The drawing under review shows one solid part. Ordinate dimensions are in mm from its lowest x, y, z. Round coordinates to 2 decimals unless told otherwise and drop trailing zeros. Write each loop counter-clockwise with the first axis right and the second up, starting at its lowest first coordinate (ties: lowest second). Pieces come first, ordered by that corner, then holes.
Item 1: Add section A-A (x = 50.8). Give the boundary of the cut face in (y, z), plus the area to 3 significant figures.
Item 2: Add section C-C (y = 14). Give the boundary of the cut face in (x, z).
Item 3: To check wall thickness, follow L1, parallel to X at y = 14.5, z = 59; L2, parallel to Z at x = 60, y = 6. State the ranges of each line that lie inside material, in increasing order.
Item 4: Clearance check with flat-ended pins moving along their axes: pin 1 Ø8 at (x, z) = (50.8, 50.8) entering from -Y; pin 2 Ø1 at (y, z) = (8, 90.5) entering from -X; pin 3 Ø10 at (y, z) = (6, 11) entering from +X; pin 4 Ø2 at (x, y) = (17.5, 10) entering from +Z. State where each tip first meets the part, or that it passes through.
Item 5: Add section B-B (z = 50.8). Give the boundary of the cut face in (x, y).
Item 6: Add section D-D (x = 7.5). Give the boundary of the cut face in (y, z), plus the area to 3 significant figures.
Item 7: Draft analysis for pull direction Z (two halves, no side actions). For the marked faces 1, 2 and 3, state which applies: +Z half, -Z half, draft (parallel to the pull), parting line (faces both ways), or undercut.
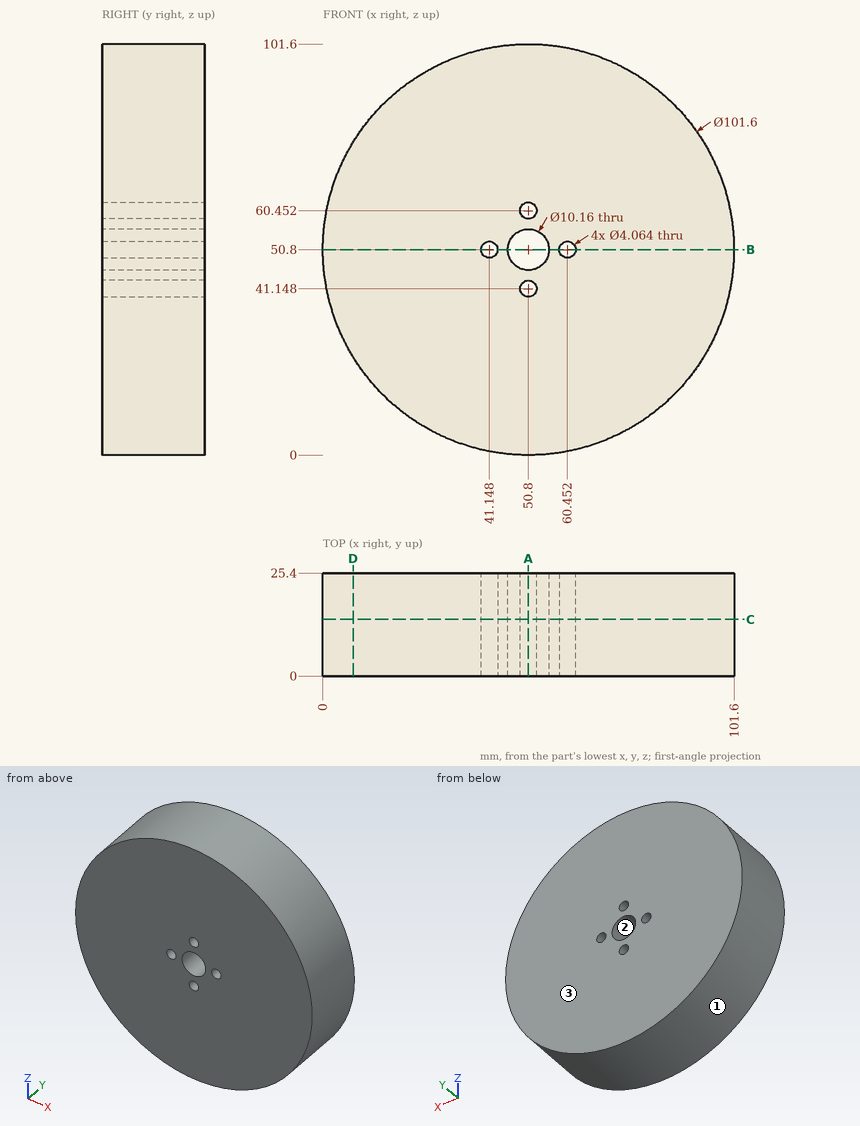
Numbers:
1. outline: (0, 0) - (25.4, 0) - (25.4, 39.12) - (0, 39.12) - close; (0, 43.18) - (25.4, 43.18) - (25.4, 45.72) - (0, 45.72) - close; (0, 55.88) - (25.4, 55.88) - (25.4, 58.42) - (0, 58.42) - close; (0, 62.48) - (25.4, 62.48) - (25.4, 101.6) - (0, 101.6) - close
1. area: 2,120 mm2
2. outline: circle Ø101.6 at (50.8, 50.8); hole circle Ø4.06 at (41.15, 50.8); hole circle Ø10.16 at (50.8, 50.8); hole circle Ø4.06 at (50.8, 41.15); hole circle Ø4.06 at (50.8, 60.45); hole circle Ø4.06 at (60.45, 50.8)
3. L1: x = 0.67 to 49.38, 52.22 to 100.93
3. L2: z = 0.84 to 48.82, 52.78 to 100.76
4. pin 1: passes through
4. pin 2: stops at x = 18.49
4. pin 3: stops at x = 87.81
4. pin 4: stops at z = 90.01
5. outline: (0, 0) - (39.12, 0) - (39.12, 25.4) - (0, 25.4) - close; (43.18, 0) - (45.72, 0) - (45.72, 25.4) - (43.18, 25.4) - close; (55.88, 0) - (58.42, 0) - (58.42, 25.4) - (55.88, 25.4) - close; (62.48, 0) - (101.6, 0) - (101.6, 25.4) - (62.48, 25.4) - close
6. outline: (0, 24.23) - (25.4, 24.23) - (25.4, 77.37) - (0, 77.37) - close
6. area: 1,350 mm2
7. face 1: parting line
7. face 2: undercut
7. face 3: draft
